Could you check a few things on this model? Use its own coordinates, in mm. Face numbers are marked on the shaded views. Give positions to 0.01 mm unless a question says otherwise; leave off trailing zeros. Loops run counter-clockwise (first coordinate to the right, second up) from the corner with the lowest first, then second, coordinate; pieces in that order, holes last. Notation, with made-up numbers: M -8.75,-14.75 L 50.25,-14.75 A24 cw 50.25,11.25 Z; hole C 88,-3.75 d10. An arc over 180 degrees is marked long. Return JSON: item names as keys, results as strings. Group by question number.
1. If we section it at C-C (x = -17.5): Write out the boundary of the cut face in (y, z).
2. Please list where these lines run through material, in increasing order: line 1 (Z direction, x = 0, y = -7.25); line 2 (Z direction, x = -2, y = 1.5); line 3 (Z direction, x = 0, y = -10.25).
3. If we section it at D-D (z = 23.25): Write out the boundary of the cut face in (x, y).
4. If we section it at A-A (x = 0): Write out the boundary of the cut face in (y, z).
5. If we mould it in two halves opening along X, with no side actions, what happens to the marked faces 1, 2 and 3? For each: +X half, -X half, draft (parallel to the pull), parting line (faces both ways), or undercut.
6. For pin 1 (6 mm diameter, centred on y = 1.5, z = 18.5, fed in from -X); pin 2 (4 mm diameter, centred on x = -30, z = 16, fed in from -Y); pin 3 (10 mm diameter, centred on x = -2.5, z = 19, fed in from +Y), each with a flat end and sliding along its axis, tell me the tip position at first contact or that it passes through.
7. If we section it at B-B (z = 8): Write out the boundary of the cut face in (x, y), plus the area to 3 significant figures.
```python
from build123d import *

# Parameters (mm, degrees)
BOSS_EXTRUDE1_DEPTH = 25
BOSS_EXTRUDE1_TAPER = 5
FILLET1_R           = 3
CUT_EXTRUDE1_DEPTH  = 0.5
BOSS_EXTRUDE2_REACH = 26.726
SKETCH5_W           = 65
SKETCH5_H           = 9
SKETCH6_R           = 2.5
CUT_EXTRUDE2_DEPTH  = 8


with BuildPart() as part:
    # Sketch1 → Boss-Extrude1 (new body)
    with BuildSketch(Plane.XY):
        with BuildLine():
            ThreePointArc((-32.5, 12.5), (-45, 0), (-32.5, -12.5))
            Line((-32.5, -12.5), (32.5, -12.5))
            ThreePointArc((32.5, -12.5), (45, 0), (32.5, 12.5))
            Line((32.5, 12.5), (-32.5, 12.5))
        make_face()
    extrude(amount=BOSS_EXTRUDE1_DEPTH, taper=BOSS_EXTRUDE1_TAPER)

    # Fillet1
    fillet1_edges = [part.edges().sort_by_distance(p)[0] for p in [
        (0, 12.5, 0),
        (45, 0, 0),
        (0, -12.5, 0),
        (-45, 0, 0),
    ]]
    fillet(fillet1_edges, radius=FILLET1_R)

    # Sketch4 → Cut-Extrude1 (cut)
    with BuildSketch(Plane.XY.offset(25)):
        with BuildLine():
            Line((-32.5, -8.812783412), (32.5, -8.812783412))
            ThreePointArc((32.5, -8.812783412), (41.312783412, 0), (32.5, 8.812783412))
            Line((32.5, 8.812783412), (-32.5, 8.812783412))
            ThreePointArc((-32.5, 8.812783412), (-41.312783412, 0), (-32.5, -8.812783412))
        make_face()
    extrude(amount=-CUT_EXTRUDE1_DEPTH, mode=Mode.SUBTRACT)

    # Sketch5 → Boss-Extrude2 (add, up to next)
    with BuildSketch(Plane(origin=(0, -12.5, 0), x_dir=(1, 0, 0), z_dir=(0, 1, 0)), mode=Mode.PRIVATE) as boss_extrude2_sk1:
        with Locations((0, -7.761467228)):
            Rectangle(SKETCH5_W, SKETCH5_H)
    boss_extrude2_tool1 = extrude(boss_extrude2_sk1.sketch, amount=BOSS_EXTRUDE2_REACH, mode=Mode.PRIVATE) - part.part
    add(boss_extrude2_tool1.solids().sort_by_distance((0, -12.5, 7.761467))[0])

    # Sketch6 → Cut-Extrude2 (cut)
    with BuildSketch(Plane.XZ.offset(12.5)):
        with Locations((0, 8)):
            Circle(SKETCH6_R)
    extrude(amount=-CUT_EXTRUDE2_DEPTH, mode=Mode.SUBTRACT)


solid = part.part
```
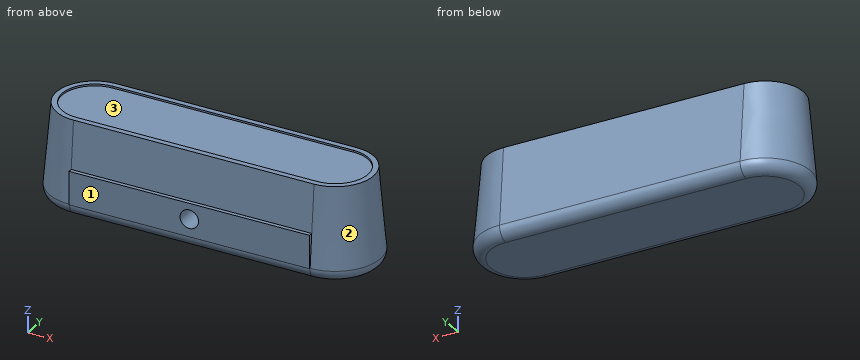
Answer:
{
 "1": {"outline": "M -12.5,3.26 L -12.21,3.26 A3 ccw -9.23,0 L 9.23,0 A3 ccw 12.21,3.26 L 10.31,25 L 8.81,25 L 8.81,24.5 L -8.81,24.5 L -8.81,25 L -10.31,25 L -11.43,12.26 L -12.5,12.26 Z"},
 "2": {"line 1": "z = 0 to 5.5, 10.5 to 24.5", "line 2": "z = 0 to 24.5", "line 3": "z = 0.18 to 5.5, 10.5 to 25"},
 "3": {"outline": "M -32.5,-10.47 L 32.5,-10.47 A10.47 ccw 32.5,10.47 L -32.5,10.47 A10.47 ccw Z"},
 "4": {"outline": "M -12.5,3.26 L -12.21,3.26 A3 ccw -9.23,0 L 9.23,0 A3 ccw 12.21,3.26 L 10.31,25 L 8.81,25 L 8.81,24.5 L -8.81,24.5 L -8.81,25 L -10.31,25 L -11.43,12.26 L -12.5,12.26 L -12.5,10.5 L -4.5,10.5 L -4.5,5.5 L -12.5,5.5 Z"},
 "5": {"face 1": "draft", "face 2": "+X half", "face 3": "undercut"},
 "6": {"pin 1": "stops at x = -43.62", "pin 2": "stops at y = -11.28", "pin 3": "stops at y = 11.28"},
 "7": {"outline": "M -32.5,-12.5 L -2.5,-12.5 L -2.5,-4.5 L 2.5,-4.5 L 2.5,-12.5 L 32.5,-12.5 L 32.5,-11.8 A11.8 ccw 32.5,11.8 L -32.5,11.8 A11.8 ccw -32.5,-11.8 Z", "area": "1,980 mm²"}
}
